Read the model definition and answer for the solid it produces. Units are mm, in the model's axes. A direction names the side the tool comes from. Round coordinates to 2 decimals unless told otherwise and drop trailing zeros. Order: outer loops, then holes, each group sorted by start corner. A loop starts at its lowest first (then second) coordinate and runs counter-clockwise, first axis right, second up. Notation, with made-up numbers: (10, 23.25) - (40, 23.25) arc R20 cw to (40, 31.25) - close; hole circle Ø2 at (71, 20). An arc over 180 degrees is marked (long way). Put each result on its own line as item: value. Start each with the question number.
Q1. Section B-B on z = 17.5 is taken. Give the vertices of the cut face in (x, y), then the cut area to 3 significant figures.
Q2. For a pull along Z with two mould halves and no side action, classify faces 4 (the face through (-13, -16, -12)), 5 (the face through (-10, 0, 11)), 6 (the face through (-2.4, -15.8, -14.3)), 7 (the face through (-19, 4.4, 2)) as pulls with the +Z half, pulls with the -Z half, needs draft (parallel to the pull), parting line crosses it, or undercut.
Q3. Each of these flat-tipped pins is pushed along its axis until it touches: pin 1 Ø10 at (x, y) = (9.5, -8) entering from -Z; pin 2 Ø4 at (x, z) = (-16.5, -1) entering from -Y. Where does it stop, or does it pass through?
Q4. Which of the six approach directions +Z, -Z, +X, -X, +Y, -Y give full straight-line access (tool end or side, diameter ignored) to faces 1 (the face through (0, -7, 24)), 2 (the face through (-20.7, 2.2, 2.4)), 3 (the face through (2.971, -15.835, -21.372))?
Q5. Find the intervals of material crossed by line 1 along X through (y, z) = (6.95, 17.5); line 2 along Y through (x, z) = (-9.5, 11.5); line 3 along Y through (x, z) = (15, 26.65), in increasing order. Write a range as from..to.
Q6. Section C-C on y = 2.25 is taken. Give the vertices of the cut face in (x, z).
Q7. Section D-D on x = 8 is taken. Give the vertices of the cut face in (y, z), then the cut area to 3 significant figures.
Q8. Section A-A on y = -7.3 is taken. Give the vertices of the cut face in (x, z).
from build123d import *

# Parameters (mm, degrees)
SKETCH_1_W               = 45
SKETCH_1_H               = 45
SKETCH_1_R               = 13
EXTRUDE_1_DEPTH          = 8
FILLET_1_R               = 20
SKETCH_2_W               = 45
SKETCH_2_H               = 8
EXTRUDE_2_DEPTH          = 6.5
PATTERN_CIRCULAR_1_COUNT = 4
SKETCH_7_W               = 45
SKETCH_7_H               = 5
EXTRUDE_3_DEPTH          = 13.3
SKETCH_9_W               = 45
SKETCH_9_H               = 5
EXTRUDE_4_DEPTH          = 51.5
SKETCH_10_R              = 13.025
CUT_EXTRUDE_1_DEPTH      = 53.3
CUT_EXTRUDE_2_REACH      = 47.155
SKETCH_11_R              = 4
HOLE_WIZARD_M4_1_2_D     = 3.3
HOLE_WIZARD_M4_1_2_DEPTH = 11.5
HOLE_WIZARD_M4_1_2_TIP   = 0.991420021
CUT_EXTRUDE_3_REACH      = 47.155
FILLET_4_R               = 10


with BuildPart() as part:
    # 草图1 → 凸台-拉伸1 (new body)
    with BuildSketch(Plane(origin=(0, 0, 0), x_dir=(1, 0, 0), z_dir=(0, 1, 0))):
        Rectangle(SKETCH_1_W, SKETCH_1_H)
        with Locations(Location((0, 0, 0), (0, 0, 270))):
            Circle(SKETCH_1_R, mode=Mode.SUBTRACT)
    extrude(amount=EXTRUDE_1_DEPTH)

    # 圆角1
    fillet_1_edges = [part.edges().sort_by_distance(p)[0] for p in [
        (-22.5, 4, -22.5),
        (22.5, 4, -22.5),
    ]]
    fillet(fillet_1_edges, radius=FILLET_1_R)

    # 草图2 → 凸台-拉伸2 (add)
    with BuildSketch(Plane.XY.offset(22.5)):
        with Locations((0, 4)):
            Rectangle(SKETCH_2_W, SKETCH_2_H)
    extrude(amount=EXTRUDE_2_DEPTH)

    # 草图6 → Hole Wizard M4 _1 (revolve, cut)
    with BuildSketch(Plane(origin=(0, 0, 17.5), x_dir=(0, 0, -1), z_dir=(1, 0, 0))):
        Polygon((0, 0), (0, 21.351936393), (2.25, 20), (2.25, 4.4), (4, 4.4), (4, 0), align=None)
    hole_wizard_m4_1 = revolve(axis=Axis((0, -6.35, 17.5), (0, 1, 0)), mode=Mode.SUBTRACT)

    # 阵列(圆周)1: Hole Wizard M4 _1 ×4 about axis
    pattern_circular_1_axis = Axis((0, 0, 0), (0, 1, 0))
    for i in range(1, PATTERN_CIRCULAR_1_COUNT):
        add(hole_wizard_m4_1.rotate(pattern_circular_1_axis, i * 360 / PATTERN_CIRCULAR_1_COUNT), mode=Mode.SUBTRACT)

    # 草图7 → 凸台-拉伸3 (add)
    with BuildSketch(Plane.XZ):
        with Locations((0, 26.5)):
            Rectangle(SKETCH_7_W, SKETCH_7_H)
    extrude(amount=EXTRUDE_3_DEPTH)

    # 草图9 → 凸台-拉伸4 (add)
    with BuildSketch(Plane.XY.offset(29)):
        with Locations((0, -15.8)):
            Rectangle(SKETCH_9_W, SKETCH_9_H)
    extrude(amount=-EXTRUDE_4_DEPTH)

    # 草图10 → 切除-拉伸1 (cut)
    with BuildSketch(Plane(origin=(0, -13.3, 0), x_dir=(1, 0, 0), z_dir=(0, 1, 0))):
        with Locations(Location((0, 0, 0), (0, 0, 270))):
            Circle(SKETCH_10_R)
    extrude(amount=-CUT_EXTRUDE_1_DEPTH, mode=Mode.SUBTRACT)

    # 草图11 → 切除-拉伸2 (cut, up to next)
    with BuildSketch(Plane(origin=(0, -18.3, 0), x_dir=(-1, 0, 0), z_dir=(0, -1, 0)), mode=Mode.PRIVATE) as cut_extrude_2_sk1:
        with Locations(Location((0, -17.5, 0), (0, 0, 90))):
            Circle(SKETCH_11_R)
    cut_extrude_2_tool1 = extrude(cut_extrude_2_sk1.sketch, amount=-CUT_EXTRUDE_2_REACH, mode=Mode.PRIVATE) & part.part
    # 草图11 → 切除-拉伸2 (cut, up to next)
    with BuildSketch(Plane(origin=(0, -18.3, 0), x_dir=(-1, 0, 0), z_dir=(0, -1, 0)), mode=Mode.PRIVATE) as cut_extrude_2_sk2:
        with Locations(Location((-17.5, 0, 0), (0, 0, 90))):
            Circle(SKETCH_11_R)
    cut_extrude_2_tool2 = extrude(cut_extrude_2_sk2.sketch, amount=-CUT_EXTRUDE_2_REACH, mode=Mode.PRIVATE) & part.part
    # 草图11 → 切除-拉伸2 (cut, up to next)
    with BuildSketch(Plane(origin=(0, -18.3, 0), x_dir=(-1, 0, 0), z_dir=(0, -1, 0)), mode=Mode.PRIVATE) as cut_extrude_2_sk3:
        with Locations(Location((0, 17.5, 0), (0, 0, 90))):
            Circle(SKETCH_11_R)
    cut_extrude_2_tool3 = extrude(cut_extrude_2_sk3.sketch, amount=-CUT_EXTRUDE_2_REACH, mode=Mode.PRIVATE) & part.part
    # 草图11 → 切除-拉伸2 (cut, up to next)
    with BuildSketch(Plane(origin=(0, -18.3, 0), x_dir=(-1, 0, 0), z_dir=(0, -1, 0)), mode=Mode.PRIVATE) as cut_extrude_2_sk4:
        with Locations(Location((17.5, 0, 0), (0, 0, 90))):
            Circle(SKETCH_11_R)
    cut_extrude_2_tool4 = extrude(cut_extrude_2_sk4.sketch, amount=-CUT_EXTRUDE_2_REACH, mode=Mode.PRIVATE) & part.part
    add(cut_extrude_2_tool1.solids().sort_by_distance((0, -18.3, 17.5))[0], mode=Mode.SUBTRACT)
    add(cut_extrude_2_tool2.solids().sort_by_distance((17.5, -18.3, 0))[0], mode=Mode.SUBTRACT)
    add(cut_extrude_2_tool3.solids().sort_by_distance((0, -18.3, -17.5))[0], mode=Mode.SUBTRACT)
    add(cut_extrude_2_tool4.solids().sort_by_distance((-17.5, -18.3, 0))[0], mode=Mode.SUBTRACT)

    # Hole Wizard M4 _1 2
    with Locations(Plane(origin=(15, -7.3, 24), x_dir=(-1, 0, 0), z_dir=(0, 0, -1))):
        with Locations((0, 0), (30, 0)):
            Hole(HOLE_WIZARD_M4_1_2_D / 2, depth=HOLE_WIZARD_M4_1_2_DEPTH)
            with Locations((0, 0, -(HOLE_WIZARD_M4_1_2_DEPTH + HOLE_WIZARD_M4_1_2_TIP / 2))):  # 118° drill point
                Cone(0, HOLE_WIZARD_M4_1_2_D / 2, HOLE_WIZARD_M4_1_2_TIP, mode=Mode.SUBTRACT)

    # 草图23 → 切除-拉伸3 (cut, up to next)
    with BuildSketch(Plane.XZ.offset(18.3), mode=Mode.PRIVATE) as cut_extrude_3_sk1:
        Polygon((-22.5, -2.5), (-2.5, -22.5), (-22.5, -22.5), align=None)
    cut_extrude_3_tool1 = extrude(cut_extrude_3_sk1.sketch, amount=-CUT_EXTRUDE_3_REACH, mode=Mode.PRIVATE) & part.part
    # 草图23 → 切除-拉伸3 (cut, up to next)
    with BuildSketch(Plane.XZ.offset(18.3), mode=Mode.PRIVATE) as cut_extrude_3_sk2:
        Polygon((22.5, -22.5), (22.5, -2.5), (2.5, -22.5), align=None)
    cut_extrude_3_tool2 = extrude(cut_extrude_3_sk2.sketch, amount=-CUT_EXTRUDE_3_REACH, mode=Mode.PRIVATE) & part.part
    add(cut_extrude_3_tool1.solids().sort_by_distance((-15.833333, -18.3, -15.833333))[0], mode=Mode.SUBTRACT)
    add(cut_extrude_3_tool2.solids().sort_by_distance((15.833333, -18.3, -15.833333))[0], mode=Mode.SUBTRACT)

    # 圆角4
    # the kernel refuses this fillet: 10 mm, written as the material it takes off along each edge
    with BuildSketch(Plane(origin=(-22.5, -28.655339059, -2.5), x_dir=(0, 0, 1), z_dir=(0, 1, 0)), Plane(origin=(-2.5, -28.655339059, -22.5), x_dir=(-0.7071067811865476, 0, 0.7071067811865476), z_dir=(0, 1, 0))) as fillet_4_piece_1:
        with BuildLine():
            CenterArc((FILLET_4_R * 0.414213562373, FILLET_4_R), FILLET_4_R, 225, 45)
            Line((-FILLET_4_R * 0.292893218813, FILLET_4_R * 0.292893218813), (0, 0))
            Line((0, 0), (FILLET_4_R * 0.414213562373, 0))
        make_face()
    extrude(amount=25.710678119, mode=Mode.SUBTRACT)
    with BuildSketch(Plane(origin=(22.5, -28.655339059, -2.5), x_dir=(0, 0, 1), z_dir=(0, 1, 0)), Plane(origin=(2.5, -28.655339059, -22.5), x_dir=(0.7071067811865476, 0, 0.7071067811865476), z_dir=(0, 1, 0))) as fillet_4_piece_2:
        with BuildLine():
            CenterArc((FILLET_4_R * 0.414213562373, -FILLET_4_R), FILLET_4_R, 90, 45)
            Line((-FILLET_4_R * 0.292893218813, -FILLET_4_R * 0.292893218813), (0, 0))
            Line((0, 0), (FILLET_4_R * 0.414213562373, 0))
        make_face()
    extrude(amount=25.710678119, mode=Mode.SUBTRACT)


solid = part.part
Findings:
1. outline: (-22.5, -18.3) - (-4, -18.3) - (-4, -13.3) - (-22.5, -13.3) - close; (-22.5, 0) - (-4, 0) - (-4, 4.4) - (-2.25, 4.4) - (-2.25, 8) - (-22.5, 8) - close; (2.25, 4.4) - (4, 4.4) - (4, 0) - (22.5, 0) - (22.5, 8) - (2.25, 8) - close; (4, -18.3) - (22.5, -18.3) - (22.5, -13.3) - (4, -13.3) - close
1. area: 494 mm2
2. face 4: pulls with the -Z half
2. face 5: needs draft
2. face 6: undercut
2. face 7: undercut
3. pin 1: z = 24
3. pin 2: y = 4.4
4. face 1: -Z, +X, -X
4. face 2: -Y
4. face 3: -Z, +X, -Y
5. line 1: -22.5..-2.25, 2.25..22.5
5. line 2: -18.3..-13.3, 0..8
5. line 3: -18.3..-8.95, -5.65..8
6. outline: (-22.5, -2.5) arc R20 ccw to (-2.5, -22.5) - (2.5, -22.5) arc R20 ccw to (22.5, -2.5) - (22.5, 29) - (-22.5, 29) - close; hole circle Ø8 at (-17.5, 0); hole circle Ø26 at (0, 0); hole circle Ø8 at (0, -17.5); hole circle Ø8 at (0, 17.5); hole circle Ø8 at (17.5, 0)
7. outline: (-18.3, -17) - (-13.3, -17) - (-13.3, -10.28) - (-18.3, -10.28) - close; (-18.3, 10.28) - (-13.3, 10.28) - (-13.3, 24) - (0, 24) - (0, 10.25) - (8, 10.25) - (8, 29) - (-18.3, 29) - close; (0, -21.73) - (8, -21.73) - (8, -10.25) - (0, -10.25) - close
7. area: 436 mm2
8. outline: (-22.5, 24) - (-16.65, 24) - (-16.65, 29) - (-22.5, 29) - close; (-13.35, 24) - (13.35, 24) - (13.35, 29) - (-13.35, 29) - close; (16.65, 24) - (22.5, 24) - (22.5, 29) - (16.65, 29) - close
